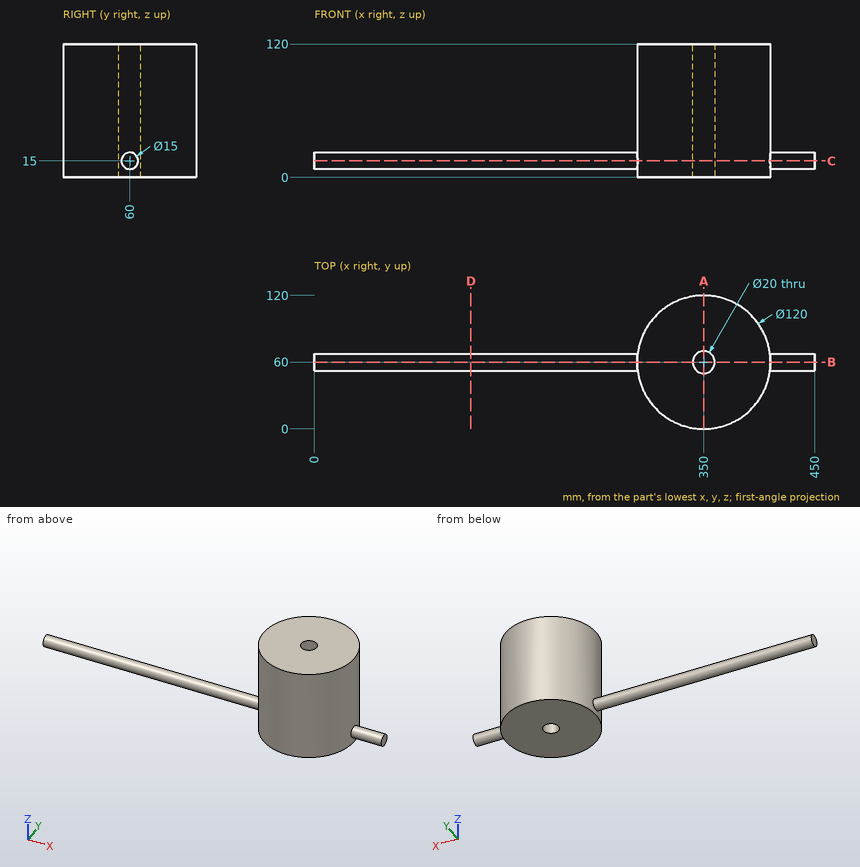
Study the drawing (mm; zero at the part's minimum x, y, z) and answer. Give positions to 0.01 mm unless a question says otherwise; leave off trailing zeros. Write each loop counter-clockwise with the first axis right and the second up, starting at its lowest first coordinate (ties: lowest second). Pieces come first, ordered by that corner, then holes. Notation, with made-up numbers: (73.25, 85) -> (112.25, 85) arc R17 ccw to (112.25, 102) -> close; hole circle Ø3 at (-2.5, -38). An arc over 180 degrees is marked (long way). Write item = value, one per line.
Q1. Section D-D on x = 140.5 is taken. Determine the outline of the cut face in (y, z).
Computed values:
outline = circle Ø15 at (60, 15)
Q2. Section C-C on z = 15 is taken. Determine the outline of the cut face in (x, y), and give its area (3 significant figures).
Computed values:
outline = (0, 52.5) -> (290.47, 52.5) arc R60 ccw to (409.53, 52.5) -> (450, 52.5) -> (450, 67.5) -> (409.53, 67.5) arc R60 ccw to (290.47, 67.5) -> (0, 67.5) -> close; hole circle Ø20 at (350, 60)
area = 16,000 mm^2
Q3. Section B-B on y = 60 is taken. Determine the outline of the cut face in (x, z).
Computed values:
outline = (0, 7.5) -> (290, 7.5) -> (290, 0) -> (340, 0) -> (340, 120) -> (290, 120) -> (290, 22.5) -> (0, 22.5) -> close; (360, 0) -> (410, 0) -> (410, 7.5) -> (450, 7.5) -> (450, 22.5) -> (410, 22.5) -> (410, 120) -> (360, 120) -> close
Q4. Section A-A on x = 350 is taken. Determine the outline of the cut face in (y, z).
Computed values:
outline = (0, 0) -> (50, 0) -> (50, 120) -> (0, 120) -> close; (70, 0) -> (120, 0) -> (120, 120) -> (70, 120) -> close
Q5. Consider line 1 along Y through (x, z) = (350, 46.5); line 2 along Z through (x, y) = (118, 61); line 3 along Y through (x, z) = (347, 44). Determine where each line is inside the solid, lowest interval first.
Computed values:
line_1 = 0 to 50, 70 to 120
line_2 = 7.57 to 22.43
line_3 = 0.08 to 50.46, 69.54 to 119.92
Q6. Flat-ended cylindrical pins translate along their axes: pin 1 Ø1 at (y, z) = (70, 62) entering from -X; pin 2 Ø12 at (y, z) = (92, 84) entering from +X; pin 3 Ø3 at (x, z) = (105.5, 12.5) entering from +Y; pin 4 Ø23 at (x, y) = (350, 60) entering from +Z. Find the tip coordinate at first contact, or state that the pin passes through.
Computed values:
pin_1 = 290.76
pin_2 = 404.07
pin_3 = 67.43
pin_4 = 120
